```python
from build123d import *

# Parameters (mm, degrees)
SKETCH1_W           = 5.5
SKETCH1_H           = 6.9
BOSS_EXTRUDE1_DEPTH = 3.2
SKETCH4_R           = 2.1
BOSS_EXTRUDE2_DEPTH = 2.1
FILLET1_R           = 2.1
SKETCH5_W           = 5.08
SKETCH5_H           = 2.78
BOSS_EXTRUDE3_DEPTH = 0.6
SKETCH7_W           = 0.5
SKETCH7_H           = 0.4
BOSS_EXTRUDE5_DEPTH = 3.19
LPATTERN1_COUNT     = 2
LPATTERN1_PITCH     = 2.54
LPATTERN1_COL_COUNT = 2
LPATTERN1_COL_PITCH = 2.54


with BuildPart() as part:
    # Sketch1 → Boss-Extrude1 (new body)
    with BuildSketch(Plane.XY):
        with Locations((2.75, 3.45)):
            Rectangle(SKETCH1_W, SKETCH1_H)
    extrude(amount=BOSS_EXTRUDE1_DEPTH)

    # Sketch4 → Boss-Extrude2 (add)
    with BuildSketch(Plane.XY.offset(3.2)):
        with Locations(Location((2.75, 4.1, 0), (0, 0, 180))):
            Circle(SKETCH4_R)
    extrude(amount=BOSS_EXTRUDE2_DEPTH)

    # Fillet1
    fillet1_edges = [part.edges().sort_by_distance(p)[0] for p in [
        (4.85, 4.1, 5.3),
    ]]
    fillet(fillet1_edges, radius=FILLET1_R - 0.0001)  # a hair under: the kernel refuses the full size

    # Sketch5 → Boss-Extrude3 (add)
    with BuildSketch(Plane.XZ):
        with Locations((2.75, 1.6)):
            Rectangle(SKETCH5_W, SKETCH5_H)
    extrude(amount=BOSS_EXTRUDE3_DEPTH)

    # Sketch7 → Boss-Extrude5 (add)
    with BuildSketch(Plane.XZ.offset(0.6)):
        with Locations((2.75, 1.6)):
            Rectangle(SKETCH7_W, SKETCH7_H)
    boss_extrude5 = extrude(amount=BOSS_EXTRUDE5_DEPTH)

    # LPattern1: Boss-Extrude5 ×2
    with Locations(*[(-i * LPATTERN1_PITCH, 0, 0) for i in range(1, LPATTERN1_COUNT)]):
        add(boss_extrude5)

    # LPattern1 col: Boss-Extrude5 ×2
    with Locations(*[(i * LPATTERN1_COL_PITCH, 0, 0) for i in range(1, LPATTERN1_COL_COUNT)]):
        add(boss_extrude5)


solid = part.part
```
The listing builds one solid part. Answer for the finished solid, in the listing's coordinates (mm). Give positions to 0.01 mm unless a question says otherwise; leave off trailing zeros. Order: outer loops, then holes, each group sorted by start corner. A loop starts at its lowest first (then second) coordinate and runs counter-clockwise, first axis right, second up. Notation, with made-up numbers: (60.25, 60.5) -> (105.25, 60.5) arc R24 cw to (105.25, 96.5) -> close; hole circle Ø3 at (78.5, 49.5). An arc over 180 degrees is marked (long way). Write each question's results on one line, items separated by ' | '.
Q1. Determine the mould class of faces 1 (the face through (3, 3, 0)), 2 (the face through (3, 6.9, 2)) for opening direction Y: pulls with the +Y half, pulls with the -Y half, needs draft (parallel to the pull), parting line crosses it, or undercut.
Checked values:
face 1: needs draft | face 2: pulls with the +Y half
Q2. The part is cut by section A-A, the plane y = -1. Give the vertices of the cut face in (x, z).
Checked values:
outline: (-0.04, 1.4) -> (0.46, 1.4) -> (0.46, 1.8) -> (-0.04, 1.8) -> close; (2.5, 1.4) -> (3, 1.4) -> (3, 1.8) -> (2.5, 1.8) -> close; (5.04, 1.4) -> (5.54, 1.4) -> (5.54, 1.8) -> (5.04, 1.8) -> close
Q3. Straight lines are drawn through the part: probe 1 along X at (y, z) = (-1.5, 1.75); probe 2 along Z at (x, y) = (0.8, -0.5); probe 3 along Z at (x, y) = (1.05, 5.75). For each, find the intervals that lie inside material, in ascending order. Write a range as from..to.
Checked values:
probe 1: x = -0.04..0.46, 2.5..3, 5.04..5.54 | probe 2: z = 0.21..2.99 | probe 3: z = 0..3.2
Q4. Each of these flat-tipped pins is pushed along its axis until it touches: P1, Ø0.7, axis at x = 3, y = -0.5, coming from the +Z side; P2, Ø1.5, axis at x = 2.5, z = 4, coming from the +Y side; P3, Ø0.7, axis at x = 2.5, y = -0.5, coming from the -Z side. Where does it stop, or does it pass through?
Checked values:
P1: stops at z = 2.99 | P2: stops at y = 6.2 | P3: stops at z = 0.21
Q5. The part is cut by section C-C, the plane z = 2.5. Give the vertices of the cut face in (x, y).
Checked values:
outline: (0, 0) -> (0.21, 0) -> (0.21, -0.6) -> (5.29, -0.6) -> (5.29, 0) -> (5.5, 0) -> (5.5, 6.9) -> (0, 6.9) -> close
Q6. The part is cut by section B-B, the plane x = 5.15. Give the vertices of the cut face in (y, z), and give its area (3 significant figures).
Checked values:
outline: (-3.79, 1.4) -> (-0.6, 1.4) -> (-0.6, 0.21) -> (0, 0.21) -> (0, 0) -> (6.9, 0) -> (6.9, 3.2) -> (0, 3.2) -> (0, 2.99) -> (-0.6, 2.99) -> (-0.6, 1.8) -> (-3.79, 1.8) -> close | area: 25.0 mm^2
